Geometry check sheet. Reference: drawing and pictorial views, mm from the part's lowest x, y, z. A direction names the side the tool comes from. Coordinates: 2 decimals unless noted, no trailing zeros. Write each loop counter-clockwise with the first axis right and the second up, starting at its lowest first coordinate (ties: lowest second). Pieces come first, ordered by that corner, then holes. Notation, with made-up numbers: (88, -20) -> (96, -20) arc R3 ccw to (96, -15) -> close; hole circle Ø4 at (74.5, -32). An arc over 180 degrees is marked (long way). Use a Markdown table: item, result.
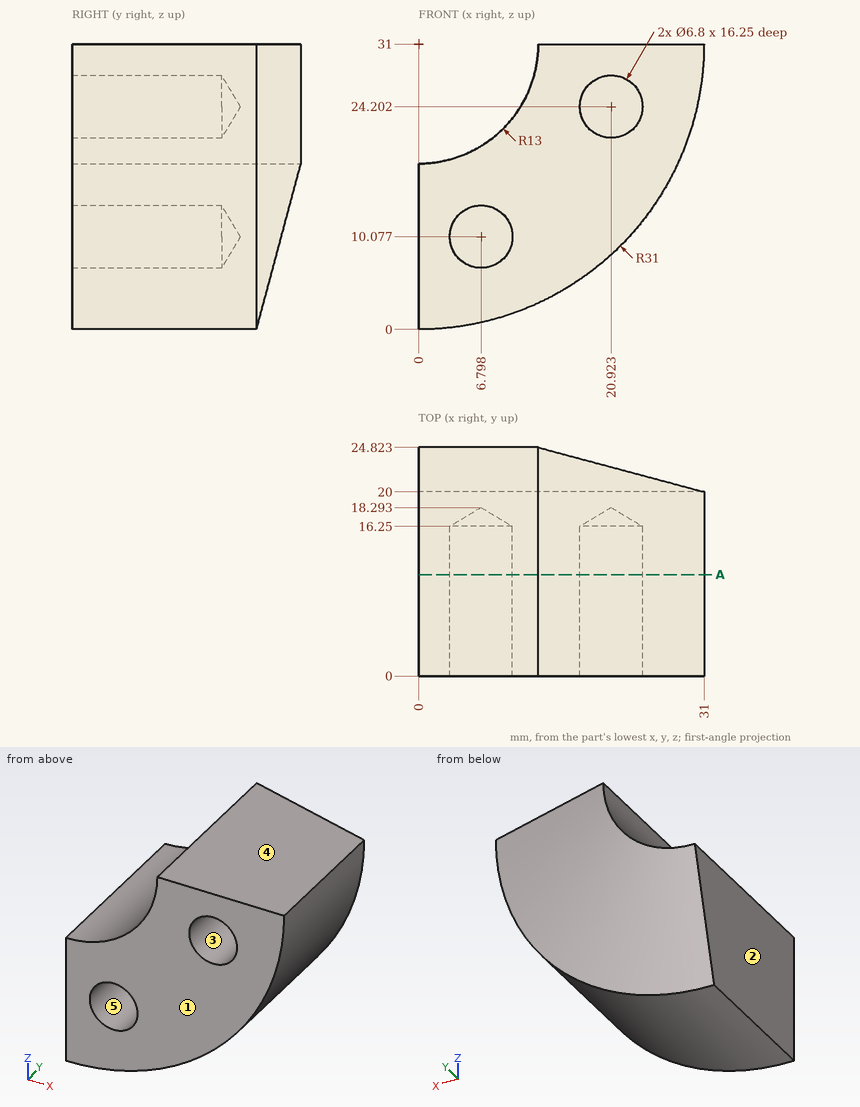
Item 1: Tool access check on the marked faces 4 and 5. Record the directions out of +Z, -Z, +X, -X, +Y, -Y that give a thin tool (end or side, any length) a straight path to the whole face; none if there is none.
Answer block:
| item | result |
|---|---|
| face 4 | +Z, +X, -X, +Y, -Y |
| face 5 | -Y |
Item 2: Depth check by flat-ended pin: P1, Ø8, axis at x = 23.5, z = 21, coming from the +Y side (1 decimal); P2, Ø5.5, axis at x = 6.8, z = 10.08, coming from the +Y side; P3, Ø6, axis at x = 7.5, z = 11, coming from the -Y side; P4, Ø1.5, axis at y = 20.5, z = 20, coming from the -X side. Enter the tip coordinate at first touch or a pass-through.
Answer block:
| item | result |
|---|---|
| P1 | stops at y = 22.5 |
| P2 | stops at y = 23.15 |
| P3 | stops at y = 0 |
| P4 | stops at x = 5.56 |
Item 3: Section check A-A on y = 11. Record the boundary of the cut face in (x, z).
Answer block:
| item | result |
|---|---|
| outline | (0, 0) arc R31 ccw to (31, 31) -> (13, 31) arc R13 cw to (0, 18) -> close; hole circle Ø6.8 at (6.8, 10.08); hole circle Ø6.8 at (20.92, 24.2) |
Item 4: Mould release check, pull along X, two halves, no side actions. Record for the marked faces 1, 2 and 3: +X half, -X half, draft (parallel to the pull), parting line (faces both ways), or undercut.
Answer block:
| item | result |
|---|---|
| face 1 | draft |
| face 2 | -X half |
| face 3 | undercut |
Item 5: Thickness scan on L1, parallel to X at y = 3.75, z = 12 (1 decimal); L2, parallel to Z at x = 21.5, y = 12.25; L3, parallel to X at y = 7.5, z = 13 (1 decimal). Record the ranges inside material, lowest first. Write a range as [from, to].
Answer block:
| item | result |
|---|---|
| L1 | x = [0, 4], [9.6, 24.5] |
| L2 | z = [8.67, 20.85], [27.55, 31] |
| L3 | x = [0, 5.1], [8.5, 25.2] |
